Can you work these out from the model? Positions are in its coordinate system, mm. A direction names the side the tool comes from. Round coordinates to 2 decimals unless told otherwise and drop trailing zeros. Order: outer loops, then holes, each group sorted by start corner. A loop starts at its lowest first (then second) coordinate and runs counter-clockwise, first axis right, second up.
from build123d import *

# Parameters (mm, degrees)
ESBO_O1_W                = 1.5
ESBO_O1_H                = 6
RESSALTO_EXTRUS_O1_DEPTH = 5
FILETE1_R                = 0.5
RESSALTO_EXTRUS_O2_DEPTH = 5


with BuildPart() as part:
    # Esboço1 → Ressalto-extrusão1 (new body)
    with BuildSketch(Plane.XY):
        with Locations((-3.25, -34.87037037)):
            Rectangle(ESBO_O1_W, ESBO_O1_H)
        with Locations((-1.75, -34.87037037)):
            Rectangle(ESBO_O1_W, ESBO_O1_H)
    extrude(amount=RESSALTO_EXTRUS_O1_DEPTH)

    # Filete1
    filete1_edges = [part.edges().sort_by_distance(p)[0] for p in [
        (-1, -31.87037037, 2.5),
        (-4, -31.87037037, 2.5),
    ]]
    fillet(filete1_edges, radius=FILETE1_R)

    # Esboço1<5> → Ressalto-extrusão2 (add, through all)
    with BuildSketch(Plane.XY):
        with BuildLine():
            Line((-4.301867323, -37.87037037), (-4, -37.87037037))
            Line((-4, -37.87037037), (-4, -37.568503047))
            ThreePointArc((-4, -37.568503047), (-4.088414892, -37.781955478), (-4.301867323, -37.87037037))
        make_face()
        with BuildLine():
            Line((-1, -37.568503047), (-1, -37.87037037))
            Line((-1, -37.87037037), (-0.698132677, -37.87037037))
            ThreePointArc((-0.698132677, -37.87037037), (-0.911585108, -37.781955478), (-1, -37.568503047))
        make_face()
    extrude(amount=RESSALTO_EXTRUS_O2_DEPTH)


solid = part.part
(1) I want a section at A-A, the plane z = 3.4. List the corners of the cut face in (x, y) for me.
(2) I'm going to push flat-ended pins straight in: pin 1 Ø2 at (y, z) = (-34, 3) entering from +X; pin 2 Ø2.5 at (y, z) = (-34, 3) entering from -X. Where does each tip first touch, or does it pass through?
(3) On a 3-axis mill with a long thin cutter (end or side, diameter ignored), from which of +Z, -Z, +X, -X, +Y, -Y can I reach the whole of each face in a straight line? I mean faces 1 (the face through (-1, -35, 2)), 2 (the face through (-3, -37.87, 2)), 3 (the face through (-4, -35, 2)). Say none if no direction works.
(4) Please list where these lines run through material, in increasing order: probe 1 along X at (y, z) = (-33.5, 1.75); probe 2 along Y at (x, z) = (-1.35, 2.95); probe 3 along Y at (x, z) = (-1.15, 3.6).
(5) I want a section at C-C, the plane x = -3.85. List the corners of the cut face in (y, z) for me, plus the area to 3 significant figures.
(6) I want a section at B-B, the plane y = -34. List the corners of the cut face in (x, z) for me.
Ans:
1. outline: (-4.3, -37.87) - (-0.7, -37.87) arc R0.3 cw to (-1, -37.57) - (-1, -32.37) arc R0.5 ccw to (-1.5, -31.87) - (-3.5, -31.87) arc R0.5 ccw to (-4, -32.37) - (-4, -37.57) arc R0.3 cw to start
2. pin 1: stops at x = -1
2. pin 2: stops at x = -4
3. face 1: +Z, -Z, +X, +Y
3. face 2: +Z, -Z, +X, -X, -Y
3. face 3: +Z, -Z, -X, +Y
4. probe 1: x = -4 to -1
4. probe 2: y = -37.87 to -31.89
4. probe 3: y = -37.87 to -32.01
5. outline: (-37.87, 0) - (-32.01, 0) - (-32.01, 5) - (-37.87, 5) - close
5. area: 29.3 mm2
6. outline: (-4, 0) - (-1, 0) - (-1, 5) - (-4, 5) - close
